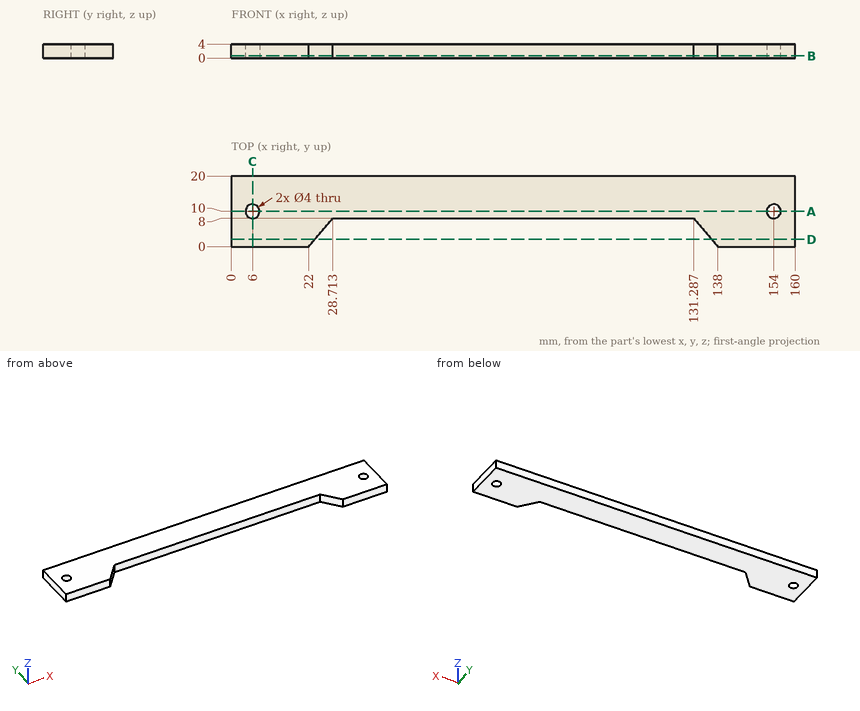
Here's the drawing with two shaded views (mm, measured from the low corner). I have some questions. Coordinates: 2 decimals unless noted, no trailing zeros. Loops run counter-clockwise (first coordinate to the right, second up) from the corner with the lowest first, then second, coordinate; pieces in that order, holes last. Notation, with made-up numbers: (59.25, 72.5) -> (64.25, 72.5) arc R31 ccw to (64.25, 105.5) -> close; hole circle Ø3 at (-13, 77.25). An arc over 180 degrees is marked (long way). Put each result on its own line as item: value. Start each with the question number.
Q1. I want a section at C-C (x = 6). Write out the boundary of the cut face in (y, z).
Q2. I want a section at B-B (z = 0.65). Write out the boundary of the cut face in (x, y), plus the area to 3 significant figures.
Q3. I want a section at A-A (y = 10). Write out the boundary of the cut face in (x, z), plus the area to 3 significant figures.
Q4. I want a section at D-D (y = 2). Write out the boundary of the cut face in (x, z), plus the area to 3 significant figures.
Q5. If I drill on line 1 (Y direction, x = 6, z = 3.15); line 2 (X direction, y = 11, z = 1.7); line 3 (Y direction, x = 81.5, z = 1.8), over which ranges is the centre line in solid material (lowest first)? Write a range as [from, to].
Taken from the geometry:
1. outline: (0, 0) -> (8, 0) -> (8, 4) -> (0, 4) -> close; (12, 0) -> (20, 0) -> (20, 4) -> (12, 4) -> close
2. outline: (0, 0) -> (22, 0) -> (28.71, 8) -> (131.29, 8) -> (138, 0) -> (160, 0) -> (160, 20) -> (0, 20) -> close; hole circle Ø4 at (6, 10); hole circle Ø4 at (154, 10)
2. area: 2,300 mm2
3. outline: (0, 0) -> (4, 0) -> (4, 4) -> (0, 4) -> close; (8, 0) -> (152, 0) -> (152, 4) -> (8, 4) -> close; (156, 0) -> (160, 0) -> (160, 4) -> (156, 4) -> close
3. area: 608 mm2
4. outline: (0, 0) -> (23.68, 0) -> (23.68, 4) -> (0, 4) -> close; (136.32, 0) -> (160, 0) -> (160, 4) -> (136.32, 4) -> close
4. area: 189 mm2
5. line 1: y = [0, 8], [12, 20]
5. line 2: x = [0, 4.27], [7.73, 152.27], [155.73, 160]
5. line 3: y = [8, 20]
